```python
from build123d import *

# Parameters (mm, degrees)
F1_DEPTH = 15


with BuildPart() as f1:
    # F0 (on Front) → F1 (new body, symmetric)
    with BuildSketch(Plane.XZ):
        with BuildLine():
            Line((-38.451876, 20.431713), (-36.795144, 19.083667))
            ThreePointArc((-36.795144, 19.083667), (-37.212223, 23.143551), (-41.272107, 22.726473))
            Line((-41.272107, 22.726473), (-39.615376, 21.378427))
            ThreePointArc((-39.615376, 21.378427), (-38.782441, 21.611757), (-38.283626, 20.90507))
            ThreePointArc((-38.283626, 20.90507), (-38.326939, 20.653885), (-38.451876, 20.431713))
        make_face()
        with BuildLine():
            Line((-50, 2), (-45, 2))
            Line((-45, 2), (-45, 9))
            Line((-45, 9), (-36.795144, 19.083667))
            Line((-36.795144, 19.083667), (-38.451876, 20.431713))
            ThreePointArc((-38.451876, 20.431713), (-39.506983, 20.32332), (-39.615376, 21.378427))
            Line((-39.615376, 21.378427), (-41.272107, 22.726473))
            Line((-41.272107, 22.726473), (-50, 12))
            Line((-50, 12), (-50, 2))
        make_face()
        Polygon((50, -2), (50, 2), (45, 2), (-45, 2), (-50, 2), (-50, -2), align=None)
        with BuildLine():
            Line((45, 2), (50, 2))
            Line((50, 2), (50, 12))
            Line((50, 12), (41.272107, 22.726473))
            Line((41.272107, 22.726473), (39.615376, 21.378427))
            ThreePointArc((39.615376, 21.378427), (39.740312, 21.156254), (39.783626, 20.90507))
            ThreePointArc((39.783626, 20.90507), (39.28481, 20.198383), (38.451876, 20.431713))
            Line((38.451876, 20.431713), (36.795144, 19.083667))
            Line((36.795144, 19.083667), (45, 9))
            Line((45, 9), (45, 2))
        make_face()
        with BuildLine():
            Line((39.615376, 21.378427), (41.272107, 22.726473))
            ThreePointArc((41.272107, 22.726473), (37.212223, 23.143551), (36.795144, 19.083667))
            Line((36.795144, 19.083667), (38.451876, 20.431713))
            ThreePointArc((38.451876, 20.431713), (38.560268, 21.48682), (39.615376, 21.378427))
        make_face()
    extrude(amount=F1_DEPTH, both=True)


solid = f1.part
```
Geometry: final body of the model. Coordinates: model frame, mm. A direction names the side the tool comes from. Round coordinates to 2 decimals unless told otherwise and drop trailing zeros. Order: outer loops, then holes, each group sorted by start corner. A loop starts at its lowest first (then second) coordinate and runs counter-clockwise, first axis right, second up. Notation, with made-up numbers: (13.5, 15.25) -> (66.5, 15.25) arc R22 ccw to (66.5, 28.25) -> close; hole circle Ø6 at (62, -34). An arc over 180 degrees is marked (long way). Use one line per item in the form item = value. Start each with the question number.
1. Line query: probe 1 along X at (y, z) = (-5.75, 21); probe 2 along X at (y, z) = (11.25, 3.5); probe 3 along Z at (x, y) = (18, 8.5). Output: solid intervals per line, ascending.
2. Pin query (flat end, axial travel): pin 1 Ø4 at (x, y) = (9.5, -0.5) entering from +Z. Return the tip coordinate at first contact, or that it passes through.
3. Draft query along Z for faces 3 (the face through (45, 0, 6)), 4 (the face through (-50, 0, 5)), 5 (the face through (-1, 0, -2)). Return one class per face: pulls with the +Z half, pulls with the -Z half, needs draft (parallel to the pull), parting line crosses it, or undercut.
4. Cut plane A-A (z = 7). Return the cut outline in (x, y).
5. Cut plane C-C (x = 13.5). Return the cut outline in (y, z).
6. Reachability of faces 1 (the face through (40.84, -0.21, 14.11)), 2 (the face through (50, 0, 5)) from +Z, -Z, +X, -X, +Y, -Y: full face, straight path, thin tool, end or side. Return the list, or none.
7. Cut plane D-D (z = 16.75). Return the cut outline in (x, y).
8. Cut plane B-B (y = -2.75). Return the cut outline in (x, z), then the cut area to 3 significant figures.
Solution:
q1.probe_1 = -42.68 to -39.78, -38.29 to -36.15, 36.15 to 38.29, 39.78 to 42.68
q1.probe_2 = -50 to -45, 45 to 50
q1.probe_3 = -2 to 2
q2.pin_1 = 2
q3.face_3 = undercut
q3.face_4 = needs draft
q3.face_5 = pulls with the -Z half
q4.outline = (-50, -15) -> (-45, -15) -> (-45, 15) -> (-50, 15) -> close; (45, -15) -> (50, -15) -> (50, 15) -> (45, 15) -> close
q5.outline = (-15, -2) -> (15, -2) -> (15, 2) -> (-15, 2) -> close
q6.face_1 = +Y, -Y
q6.face_2 = +Z, -Z, +X, +Y, -Y
q7.outline = (-46.14, -15) -> (-38.69, -15) -> (-38.69, 15) -> (-46.14, 15) -> close; (38.69, -15) -> (46.14, -15) -> (46.14, 15) -> (38.69, 15) -> close
q8.outline = (-50, -2) -> (50, -2) -> (50, 12) -> (41.27, 22.73) arc R2.89 ccw to (36.8, 19.08) -> (45, 9) -> (45, 2) -> (-45, 2) -> (-45, 9) -> (-36.8, 19.08) arc R2.89 ccw to (-41.27, 22.73) -> (-50, 12) -> close; hole (-38.45, 20.43) arc R0.75 ccw to (-38.28, 20.91) arc R0.75 ccw (long way) to start; hole (39.62, 21.38) arc R0.75 ccw (long way) to (39.78, 20.91) arc R0.75 ccw to start
q8.area = 662 mm^2
